Design review of the part built by this model. Coordinates are the model's own, in mm. Face numbers are marked on the shaded views. A direction names the side the tool comes from. Round coordinates to 2 decimals unless told otherwise and drop trailing zeros. Order: outer loops, then holes, each group sorted by start corner. A loop starts at its lowest first (then second) coordinate and runs counter-clockwise, first axis right, second up. Notation, with made-up numbers: (6.5, -2) - (22.5, -2) arc R33 cw to (22.5, 27) - close; hole circle Ø2 at (17, 7). An arc over 180 degrees is marked (long way). Use CSV: the item, a comma, the result in double quotes.
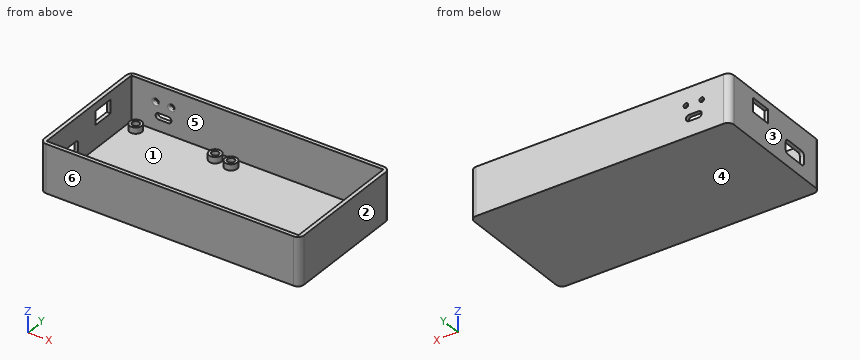
from build123d import *

# Parameters (mm, degrees)
SKETCH_1_W          = 170
SKETCH_1_H          = 85
EXTRUDE_1_DEPTH     = 2.5
SKETCH_2_W          = 170
SKETCH_2_H          = 85
SKETCH_2_W_2        = 165
SKETCH_2_H_2        = 80
EXTRUDE_1_2_DEPTH   = 29
SKETCH_3_R          = 4
EXTRUDE_2_DEPTH     = 4
SKETCH_4_R          = 2.35
CUT_EXTRUDE_1_DEPTH = 6
SKETCH_5_W          = 9.022635
SKETCH_5_H          = 17.078559106
CUT_EXTRUDE_2_DEPTH = 3
SKETCH_6_W          = 10.304284877
SKETCH_6_H          = 4.085444359
CUT_EXTRUDE_3_DEPTH = 3
FILLET_1_R          = 2
FILLET_2_R          = 2
EXTRUDE_START       = 2.5
EXTRUDE_3_OUTLINE_R = 4
EXTRUDE_3_DEPTH     = 4
SKETCH_8_R          = 2.35
CUT_EXTRUDE_4_DEPTH = 5
SKETCH_9_W          = 9
SKETCH_9_H          = 14
CUT_EXTRUDE_5_DEPTH = 5
FILLET_5_R          = 4
SKETCH_10_R         = 1.5
CUT_EXTRUDE_6_DEPTH = 5
FILLET_7_R          = 1
FILLET_8_R          = 1


# Read off the part's stored shape, not the designer's step: Бобышка-Вытянуть3
with BuildPart() as part:
    # Эскиз1 → Extrude 1 (new body)
    with BuildSketch(Plane.XY):
        Rectangle(SKETCH_1_W, SKETCH_1_H)
    extrude(amount=EXTRUDE_1_DEPTH)

    # Эскиз2 → Extrude 1 2 (add)
    with BuildSketch(Plane.XY.offset(2.5)):
        Rectangle(SKETCH_2_W, SKETCH_2_H)
        Rectangle(SKETCH_2_W_2, SKETCH_2_H_2, mode=Mode.SUBTRACT)
    extrude(amount=EXTRUDE_1_2_DEPTH)

    # Эскиз3 → Бобышка-Вытянуть2 (add)
    with BuildSketch(Plane.XY.offset(2.5)):
        with Locations((-75.5, 34)):
            Circle(SKETCH_3_R)
        with Locations((-23.5, 34)):
            Circle(SKETCH_3_R)
        with Locations((-23.5, -34)):
            Circle(SKETCH_3_R)
        with Locations((-75.5, -34)):
            Circle(SKETCH_3_R)
    extrude(amount=EXTRUDE_2_DEPTH)

    # Эскиз4 → Вырез-Вытянуть1 (cut)
    with BuildSketch(Plane.XY.offset(6.5)):
        with Locations((-75.5, 34)):
            Circle(SKETCH_4_R)
        with Locations((-23.5, 34)):
            Circle(SKETCH_4_R)
        with Locations((-75.5, -34)):
            Circle(SKETCH_4_R)
        with Locations((-23.5, -34)):
            Circle(SKETCH_4_R)
    extrude(amount=-CUT_EXTRUDE_1_DEPTH, mode=Mode.SUBTRACT)

    # Эскиз5 → Вырез-Вытянуть2 (cut)
    with BuildSketch(Plane.ZY.offset(85)):
        with Locations((12.205393393, -18.810582789)):
            Rectangle(SKETCH_5_W, SKETCH_5_H)
    extrude(amount=-CUT_EXTRUDE_2_DEPTH, mode=Mode.SUBTRACT)

    # Эскиз6 → Вырез-Вытянуть3 (cut)
    with BuildSketch(Plane(origin=(0, 42.5, 0), x_dir=(1, 0, 0), z_dir=(0, 1, 0))):
        with Locations((-61.466763375, -11.87482218)):
            Rectangle(SKETCH_6_W, SKETCH_6_H)
    extrude(amount=-CUT_EXTRUDE_3_DEPTH, mode=Mode.SUBTRACT)

    # Скругление1
    fillet_1_edges = [part.edges().sort_by_distance(p)[0] for p in [
        (-83.75, -27.349862342, 7.694075893),
        (-83.75, -10.271303236, 7.694075893),
        (-83.75, -10.271303236, 16.716710893),
        (-83.75, -27.349862342, 16.716710893),
    ]]
    fillet(fillet_1_edges, radius=FILLET_1_R)

    # Скругление2
    fillet_2_edges = [part.edges().sort_by_distance(p)[0] for p in [
        (-66.618905813, 41.25, 13.917544359),
        (-66.618905813, 41.25, 9.8321),
        (-56.314620936, 41.25, 9.8321),
        (-56.314620936, 41.25, 13.917544359),
    ]]
    fillet(fillet_2_edges, radius=FILLET_2_R)

    # Бобышка-Вытянуть3 outline → Бобышка-Вытянуть3 (add)
    with BuildSketch(Plane.XY.offset(EXTRUDE_START)):
        with Locations((-12.4283067, 32.990374872)):
            Circle(EXTRUDE_3_OUTLINE_R)
        with Locations((75.5716933, 32.990374872)):
            Circle(EXTRUDE_3_OUTLINE_R)
        with Locations((-12.4283067, -35.009625128)):
            Circle(EXTRUDE_3_OUTLINE_R)
        with Locations((75.5716933, -35.009625128)):
            Circle(EXTRUDE_3_OUTLINE_R)
    extrude(amount=EXTRUDE_3_DEPTH)

    # Эскиз8 → Вырез-Вытянуть4 (cut)
    with BuildSketch(Plane.XY.offset(6.5)):
        with Locations((-12.4283067, -35.009625128)):
            Circle(SKETCH_8_R)
        with Locations((75.5716933, -35.009625128)):
            Circle(SKETCH_8_R)
        with Locations((75.5716933, 32.990374872)):
            Circle(SKETCH_8_R)
        with Locations((-12.4283067, 32.990374872)):
            Circle(SKETCH_8_R)
    extrude(amount=-CUT_EXTRUDE_4_DEPTH, mode=Mode.SUBTRACT)

    # Эскиз9 → Вырез-Вытянуть5 (cut)
    with BuildSketch(Plane.ZY.offset(85)):
        with Locations((22.023559844, 13.353303456)):
            Rectangle(SKETCH_9_W, SKETCH_9_H)
    extrude(amount=-CUT_EXTRUDE_5_DEPTH, mode=Mode.SUBTRACT)

    # Скругление5
    fillet_5_edges = [part.edges().sort_by_distance(p)[0] for p in [
        (85, -42.5, 15.75),
        (-85, -42.5, 15.75),
        (-85, 42.5, 15.75),
        (85, 42.5, 15.75),
    ]]
    fillet(fillet_5_edges, radius=FILLET_5_R)

    # Эскиз10 → Вырез-Вытянуть6 (cut)
    with BuildSketch(Plane(origin=(0, 42.5, 0), x_dir=(1, 0, 0), z_dir=(0, 1, 0))):
        with Locations(Location((-66.618905813, -20.487054891, 0), (0, 0, 270))):
            Circle(SKETCH_10_R)
        with Locations(Location((-56.314620936, -20.487054891, 0), (0, 0, 270))):
            Circle(SKETCH_10_R)
    extrude(amount=-CUT_EXTRUDE_6_DEPTH, mode=Mode.SUBTRACT)

    # Скругление7
    fillet_7_edges = [part.edges().sort_by_distance(p)[0] for p in [
        (-56.314620936, 40, 18.987054891),
    ]]
    fillet(fillet_7_edges, radius=FILLET_7_R)

    # Скругление8
    fillet_8_edges = [part.edges().sort_by_distance(p)[0] for p in [
        (-66.618905813, 40, 18.987054891),
    ]]
    fillet(fillet_8_edges, radius=FILLET_8_R)


solid = part.part
1) We need section B-B (x = -23.5). Give the boundary of the cut face in (y, z), then the cut area to 3 significant figures.
Data:
outline,"(-42.5, 0) - (42.5, 0) - (42.5, 31.5) - (40, 31.5) - (40, 2.5) - (38, 2.5) - (38, 6.5) - (36.35, 6.5) - (36.35, 0.5) - (31.65, 0.5) - (31.65, 6.5) - (30, 6.5) - (30, 2.5) - (-30, 2.5) - (-30, 6.5) - (-31.65, 6.5) - (-31.65, 0.5) - (-36.35, 0.5) - (-36.35, 6.5) - (-38, 6.5) - (-38, 2.5) - (-40, 2.5) - (-40, 31.5) - (-42.5, 31.5) - close"
area,"365 mm2"
2) For the marked faces 5 and 6, list the 3-axis set-ups (+Z, -Z, +X, -X, +Y, -Y) from which the entire face can be reached by the end or side of a thin tool; tool diameter is ignored.
Data:
face 5,"+Z"
face 6,"+Z, -Z, +X, -X, -Y"
3) We need section A-A (y = 11). Give the boundary of the cut face in (x, z), then the cut area to 4 significant figures.
Data:
outline,"(-85, 0) - (85, 0) - (85, 31.5) - (82.5, 31.5) - (82.5, 2.5) - (-82.5, 2.5) - (-82.5, 17.52) - (-85, 17.52) - close; (-85, 26.52) - (-82.5, 26.52) - (-82.5, 31.5) - (-85, 31.5) - close"
area,"547.5 mm2"
4) We need section D-D (x = 49.5). Give the boundary of the cut face in (y, z).
Data:
outline,"(-42.5, 0) - (42.5, 0) - (42.5, 31.5) - (40, 31.5) - (40, 2.5) - (-40, 2.5) - (-40, 31.5) - (-42.5, 31.5) - close"
5) We need section C-C (y = -18.5). Give the boundary of the cut face in (x, z).
Data:
outline,"(-85, 0) - (85, 0) - (85, 31.5) - (82.5, 31.5) - (82.5, 2.5) - (-82.5, 2.5) - (-82.5, 7.69) - (-85, 7.69) - close; (-85, 16.72) - (-82.5, 16.72) - (-82.5, 31.5) - (-85, 31.5) - close"
6) To check wall thickness, follow L1, parallel to Y at x = -75.5, z = 4.8; L2, parallel to Y at x = 30, z = 21; L3, parallel to X at y = 15, z = 30.5. State the ranges of each line that lie inside material, in increasing order. Write a range as from..to.
Data:
L1,"y = -42.5..-40, -38..-36.35, -31.65..-30, 30..31.65, 36.35..38, 40..42.5"
L2,"y = -42.5..-40, 40..42.5"
L3,"x = -85..-82.5, 82.5..85"
7) Insertion check: pin 1 Ø2 at (x, y) = (-2, 10.5) entering from -Z; pin 2 Ø1.4 at (x, y) = (-23.5, -34) entering from +Z; pin 3 Ø9 at (x, y) = (-77.5, -33.5) entering from +Z; pin 4 Ø24 at (x, y) = (-20.5, -8) entering from +Z. Each pin has a flat end and moves straight along its axis. Give the tip position at first contact, or say it passes through.
Data:
pin 1,"stops at z = 0"
pin 2,"stops at z = 0.5"
pin 3,"stops at z = 6.5"
pin 4,"stops at z = 2.5"
8) The part is to be moulded in two halves that separate along X. For the marked faces 1, 2, 3 and 4, say which applies: +X half, -X half, draft (parallel to the pull), parting line (faces both ways), or undercut.
Data:
face 1,"undercut"
face 2,"+X half"
face 3,"-X half"
face 4,"draft"
